Can you work these out from the model? Positions are in its coordinate system, mm. Face numbers are marked on the shaded views. A direction names the side the tool comes from. Give positions to 0.01 mm unless a question says otherwise; leave off trailing zeros. Loops run counter-clockwise (first coordinate to the right, second up) from the corner with the lowest first, then second, coordinate; pieces in that order, holes last.
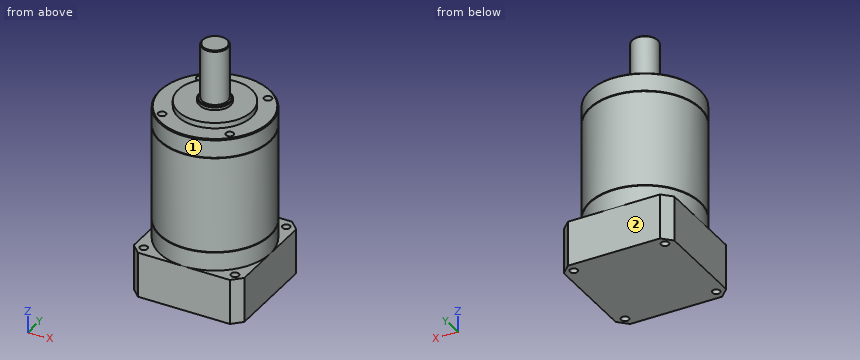
from build123d import *

# Parameters (mm, degrees)
SKETCH_1_W               = 60
SKETCH_1_H               = 60
EXTRUDE_1_DEPTH          = 24.5
CHAMFER_1_SIZE           = 5
SKETCH_2_R               = 30
EXTRUDE_2_DEPTH          = 73
SKETCH_3_W               = 0.5
SKETCH_3_H               = 3.76881343
SKETCH_4_R               = 7
EXTRUDE_3_DEPTH          = 35
SKETCH_5_R               = 20
EXTRUDE_4_DEPTH          = 3
SKETCH_6_R               = 8.5
EXTRUDE_5_DEPTH          = 2
PATTERN_CIRCULAR_1_COUNT = 4
HOLE_WIZARD_M5_2_D       = 4.2
PATTERN_CIRCULAR_2_COUNT = 4
CHAMFER_2_SIZE           = 0.5


with BuildPart() as part:
    # 草图1 → 凸台-拉伸1 (new body)
    with BuildSketch(Plane.XY):
        Rectangle(SKETCH_1_W, SKETCH_1_H)
    extrude(amount=EXTRUDE_1_DEPTH)

    # 倒角1
    chamfer_1_edges = [part.edges().sort_by_distance(p)[0] for p in [
        (30, -30, 12.25),
        (-30, -30, 12.25),
        (-30, 30, 12.25),
        (30, 30, 12.25),
    ]]
    chamfer(chamfer_1_edges, length=CHAMFER_1_SIZE)

    # 草图2 → 凸台-拉伸2 (add)
    with BuildSketch(Plane.XY.offset(24.5)):
        Circle(SKETCH_2_R)
    extrude(amount=EXTRUDE_2_DEPTH)

    # 草图3 → 切除-旋转1 (revolve, cut)
    with BuildSketch(Plane(origin=(0, 0, 0), x_dir=(0, 0, -1), z_dir=(1, 0, 0)), mode=Mode.PRIVATE) as cut_revolve_1_sk:
        with Locations((-87.25, 31.384406715)):
            Rectangle(SKETCH_3_W, SKETCH_3_H)
        with Locations((-34.75, 31.384406715)):
            Rectangle(SKETCH_3_W, SKETCH_3_H)
    revolve(cut_revolve_1_sk.sketch.rotate(Axis((0, 0, 0), (0, 0, 1)), 90), axis=Axis((0, 0, 0), (0, 0, 1)), mode=Mode.SUBTRACT)

    # 草图4 → 凸台-拉伸3 (add)
    with BuildSketch(Plane.XY.offset(97.5)):
        Circle(SKETCH_4_R)
    extrude(amount=EXTRUDE_3_DEPTH)

    # 草图5 → 凸台-拉伸4 (add)
    with BuildSketch(Plane.XY.offset(97.5)):
        Circle(SKETCH_5_R)
    extrude(amount=EXTRUDE_4_DEPTH)

    # 草图6 → 凸台-拉伸5 (add)
    with BuildSketch(Plane.XY.offset(100.5)):
        Circle(SKETCH_6_R)
    extrude(amount=EXTRUDE_5_DEPTH)

    # 草图7 → M5 螺纹孔1 (revolve, cut)
    with BuildSketch(Plane(origin=(18.384776311, 18.384776311, 97.5), x_dir=(0, -1, 0), z_dir=(1, 0, 0))):
        Polygon((0, 0), (0, 13.6618073), (2.1, 12.4), (2.1, 0), align=None)
    hole_wizard_m5_1 = revolve(axis=Axis((18.384776311, 18.384776311, 103.85), (0, 0, -1)), mode=Mode.SUBTRACT)

    # 阵列(圆周)1: M5 螺纹孔1 ×4 about axis
    pattern_circular_1_axis = Axis((0, 0, 0), (0, 0, 1))
    for i in range(1, PATTERN_CIRCULAR_1_COUNT):
        add(hole_wizard_m5_1.rotate(pattern_circular_1_axis, i * 360 / PATTERN_CIRCULAR_1_COUNT), mode=Mode.SUBTRACT)

    # M5 螺纹孔2 (through all)
    with Locations(Plane(origin=(0, 0, 0), x_dir=(-1, 0, 0), z_dir=(0, 0, -1))):
        with Locations((24.748737342, 24.748737342)):
            hole_wizard_m5_2 = Hole(HOLE_WIZARD_M5_2_D / 2)

    # 阵列(圆周)2: M5 螺纹孔2 ×4 about axis
    pattern_circular_2_axis = Axis((0, 0, 0), (0, 0, 1))
    for i in range(1, PATTERN_CIRCULAR_2_COUNT):
        add(hole_wizard_m5_2.rotate(pattern_circular_2_axis, i * 360 / PATTERN_CIRCULAR_2_COUNT), mode=Mode.SUBTRACT)

    # 倒角2
    chamfer_2_edges = [part.edges().sort_by_distance(p)[0] for p in [
        (-30, 0, 97.5),
        (-7, 0, 132.5),
        (-8.5, 0, 102.5),
    ]]
    chamfer(chamfer_2_edges, length=CHAMFER_2_SIZE)


solid = part.part
(1) Will these pins go through, and if not, where does the flat tip stop? P1, Ø6.5, axis at x = -18.38, y = 18.38, coming from the +Z side; P2, Ø1, axis at x = 15.5, y = -8, coming from the +Z side; P3, Ø1, axis at x = 10.5, z = 86.5, coming from the -Y side.
Returned:
P1: stops at z = 97.5
P2: stops at z = 100.5
P3: stops at y = -28.28
(2) Which directions (+Z, -Z, +X, -X, +Y, -Y) give clear straight access to the entire face, cutting with the end or side of a thin tool? Please do the marked faces 1 and 2.
Returned:
face 1: +Z
face 2: +Z, -Z, +X, -X, +Y
(3) Suppose I cut it at C-C on z = 71. List the corners of the cut face in (x, y) for me, plus the area to 3 significant figures.
Returned:
outline: circle Ø60 at (0, 0)
area: 2,830 mm2
(4) Suppose I cut it at B-B on z = 91. List the corners of the cut face in (x, y) for me, plus the area to 3 significant figures.
Returned:
outline: circle Ø60 at (0, 0); hole circle Ø4.2 at (-18.38, -18.38); hole circle Ø4.2 at (-18.38, 18.38); hole circle Ø4.2 at (18.38, -18.38); hole circle Ø4.2 at (18.38, 18.38)
area: 2,770 mm2
(5) Please list where these lines run through material, in increasing order: probe 1 along X at (y, z) = (5.5, 69); probe 2 along Z at (x, y) = (-12.5, 10.5); probe 3 along Z at (x, y) = (3, -21.5).
Returned:
probe 1: x = -29.49 to 29.49
probe 2: z = 0 to 100.5
probe 3: z = 0 to 97.5
(6) Suppose I cut it at A-A on z = 12. List the corners of the cut face in (x, y) for me, plus the area to 3 significant figures.
Returned:
outline: (-30, -25) - (-25, -30) - (25, -30) - (30, -25) - (30, 25) - (25, 30) - (-25, 30) - (-30, 25) - close; hole circle Ø4.2 at (-24.75, -24.75); hole circle Ø4.2 at (-24.75, 24.75); hole circle Ø4.2 at (24.75, -24.75); hole circle Ø4.2 at (24.75, 24.75)
area: 3,490 mm2
